from build123d import *

# Parameters (mm, degrees)
RESSALTO_EXTRUS_O1_DEPTH = 8
ESBO_O2_W                = 20
ESBO_O2_H                = 8
RESSALTO_EXTRUS_O2_DEPTH = 25
FILETE1_R                = 4


with BuildPart() as part:
    # Esboço1 → Ressalto-extrusão1 (new body)
    with BuildSketch(Plane(origin=(0, 0, 0), x_dir=(1, 0, 0), z_dir=(0, 1, 0))):
        with BuildLine():
            Line((0, 0), (20, 0))
            Line((20, 0), (20, 34))
            ThreePointArc((20, 34), (10, 44), (0, 34))
            Line((0, 34), (0, 0))
        make_face()
    extrude(amount=RESSALTO_EXTRUS_O1_DEPTH)

    # Esboço2 → Ressalto-extrusão2 (add)
    with BuildSketch(Plane(origin=(0, 8, 0), x_dir=(1, 0, 0), z_dir=(0, 1, 0))):
        with Locations((10, 4)):
            Rectangle(ESBO_O2_W, ESBO_O2_H)
    extrude(amount=RESSALTO_EXTRUS_O2_DEPTH)

    # Filete1
    filete1_edges = [part.edges().sort_by_distance(p)[0] for p in [
        (10, 8, -8),
        (10, 0, 0),
    ]]
    fillet(filete1_edges, radius=FILETE1_R)


solid = part.part
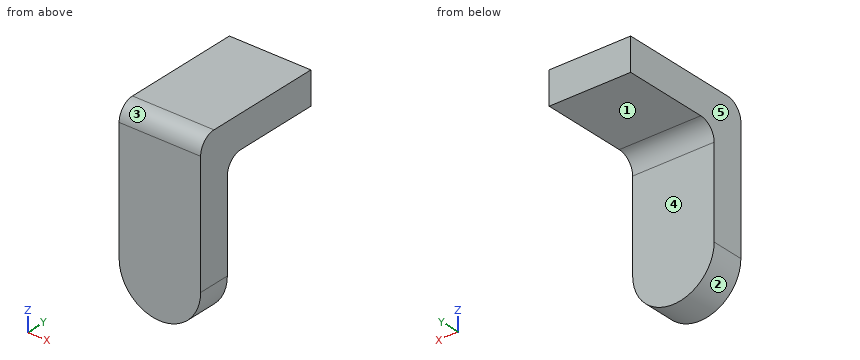
Could you check a few things on this model? Use its own coordinates, in mm. Face numbers are marked on the shaded views. A direction names the side the tool comes from. Coordinates: 2 decimals unless noted, no trailing zeros. Order: outer loops, then holes, each group sorted by start corner. A loop starts at its lowest first (then second) coordinate and runs counter-clockwise, first axis right, second up. Notation, with made-up numbers: (3.5, 68) -> (58.5, 68) arc R8 cw to (58.5, 75) -> close; hole circle Ø11 at (72.5, -33.5). An arc over 180 degrees is marked (long way). One line per item, written item: value. Start each with the question number.
1) Imagine slicing it at B-B on y = 24. List the corners of the cut face in (x, z) for me, plus the area to 3 significant figures.
2) We'd pull the mould along Y, two halves only. Please class the marked faces 3, 4 and 5: +Y half, -Y half, draft (parallel to the pull), parting line (faces both ways), or undercut.
3) Imagine slicing it at D-D on x = 10. List the corners of the cut face in (y, z) for me.
4) I'm going to push flat-ended pins straight in: pin 1 (12 mm diameter, centred on y = 26, z = -6, fed in from -X); pin 2 (2 mm diameter, centred on x = 6, z = -25.5, fed in from +Y); pin 3 (4 mm diameter, centred on x = 8, y = 25.5, fed in from -Z). Where does each tip first touch, or does it pass through?
5) Imagine slicing it at C-C on z = -26. List the corners of the cut face in (x, y) for me.
6) If I drill on L1, parallel to Z at x = 3.5, y = 18; L2, parallel to Y at x = 3.5, z = -13.5; L3, parallel to Z at x = 4.5, y = 6.5, over which ranges is the centre line in solid material (lowest first)? Write a range as [from, to].
7) Which directions (+Z, -Z, +X, -X, +Y, -Y) give clear straight access to the entire face, cutting with the end or side of a thin tool? Please do the marked faces 1 and 2.
8) Imagine slicing it at A-A on x = 16. List the corners of the cut face in (y, z) for me.
Answer list:
1. outline: (0, -8) -> (20, -8) -> (20, 0) -> (0, 0) -> close
1. area: 160 mm2
2. face 3: -Y half
2. face 4: +Y half
2. face 5: draft
3. outline: (0, -44) -> (8, -44) -> (8, -12) arc R4 cw to (12, -8) -> (33, -8) -> (33, 0) -> (4, 0) arc R4 ccw to (0, -4) -> close
4. pin 1: stops at x = 0
4. pin 2: stops at y = 8
4. pin 3: stops at z = -8
5. outline: (0, 0) -> (20, 0) -> (20, 8) -> (0, 8) -> close
6. L1: z = [-8, 0]
6. L2: y = [0, 8]
6. L3: z = [-42.35, 0]
7. face 1: -Z, +X, -X, +Y
7. face 2: -Z, +Y, -Y
8. outline: (0, -42) -> (8, -42) -> (8, -12) arc R4 cw to (12, -8) -> (33, -8) -> (33, 0) -> (4, 0) arc R4 ccw to (0, -4) -> close
